Part model, mm, in its own coordinate system. A direction names the side the tool comes from. Round coordinates to 2 decimals unless told otherwise and drop trailing zeros. Order: outer loops, then holes, each group sorted by start corner. A loop starts at its lowest first (then second) coordinate and runs counter-clockwise, first axis right, second up. Notation, with made-up numbers: M 32.5,75 L 86.5,75 A31 cw 86.5,113 Z; hole C 17,-23 d3. An arc over 180 degrees is marked long. One line per question, with ' | ' between items.
Autodesk Inventor part; units mm, degrees
ref_plane "YZ Plane" through (0, 0, 0) normal (1, 0, 0) x (0, 1, 0)
ref_plane "XZ Plane" through (0, 0, 0) normal (0, 1, 0) x (-1, 0, 0)
ref_plane "XY Plane" through (0, 0, 0) normal (0, 0, 1) x (1, 0, 0)
sketch "スケッチ1" plane through (0, 0, 0) normal (0, 1, 0) x (-1, 0, 0)
  line L0 (25, -44) -> (-25, -44)
  line L1 (-25, -44) -> (-25, 44)
  line L2 (-25, 44) -> (25, 44)
  line L3 (25, 44) -> (25, -44)
  line L4 (25, -44) -> (-25, 44) construction
  line L5 (-25, -44) -> (25, 44) construction
  point P0 (0, 0)
  dimension "d0" = 50
  dimension "d1" = 88
extrude "押し出し1" add sketch "スケッチ1" against normal blind 2
sketch "スケッチ2" plane through (0, -2, 0) normal (0, -1, 0) x (1, 0, 0)
  line L0 (-25, 44) -> (-25, -44)
  line L1 (25, -44) -> (25, 44)
  line L2 (-25, -44) -> (25, -44)
  line L3 (25, -44) -> (25, -42)
  line L4 (25, -42) -> (-25, -42)
  line L5 (-25, -42) -> (-25, -44)
  line L6 (25, 44) -> (-25, 44)
  line L7 (-25, 44) -> (25, 44)
  line L8 (25, 44) -> (25, 42)
  line L9 (25, 42) -> (-25, 42)
  line L10 (-25, 42) -> (-25, 44)
  point P0 (0, 0)
  point P1 (-25, 42)
  point P2 (25, 42)
  point P3 (25, -44)
  dimension "d4" = 2
  dimension "d5" = 2
extrude "押し出し2" add sketch "スケッチ2" along normal blind 53 contours L6 L1 L9 L0 | L4 L1 L2 L0
sketch "スケッチ3" plane through (-25, 0, 44) normal (0, 0, 1) x (1, 0, 0)
  line L0 (0, 0) -> (50, 0)
  line L1 (0, 0) -> (0, -55)
  line L2 (50, -55) -> (0, -55)
  line L3 (50, 0) -> (50, -55)
  circle A0 centre (25, -30) radius 25
  line L4 (50, 0) -> (50, -55)
  point P0 (25, 0)
  point P1 (50, -30)
  point P2 (25, -55)
  point P3 (0, -30)
extrude "押し出し3" cut sketch "スケッチ3" against normal through all contours A0 L2 L1 | L3 L2 A0
move or copy body "移動1" bodies to move or copy 1 copy no translate (0, 30, 0)
sketch "スケッチ4" plane through (-25, 28, 42) normal (0, -1, 0) x (1, 0, 0)
  circle A0 centre (25, -42) radius 34
  dimension "d14" = 68
extrude "押し出し4" add sketch "スケッチ4" against normal blind 18
fillet "フィレット2" radius 12 4 edges at (25, 29, 23.0434) (25, 29, -23.0434) (-25, 29, 23.0434) (-25, 29, -23.0434)
properties part number "link4"
1) Saw through at D-D (y = 41.5). List the corners of the cut face in (x, z), plus the area to 3 significant figures.
The answers:
outline: C 0,0 d68 | area: 3,630 mm²
2) Drop flat-ended pins along their axis: pin 1 (1.5 mm diameter, centred on x = -9.5, z = -16.5, fed in from -Y); pin 2 (13.5 mm diameter, centred on y = 15.5, z = 38.5, fed in from -X); pin 3 (7 mm diameter, centred on x = -8.5, z = 37, fed in from +Y). Give the stop position or say it passes through.
The answers:
pin 1: stops at y = 28 | pin 2: stops at x = -25 | pin 3: stops at y = 30
3) Saw through at B-B (x = 0). List the corners of the cut face in (y, z).
The answers:
outline: M -25,-44 L 30,-44 L 30,-34 L 46,-34 L 46,34 L 30,34 L 30,44 L -25,44 L -25,42 L 28,42 L 28,-42 L -25,-42 Z
4) Saw through at C-C (z = -31). List the corners of the cut face in (x, y), plus the area to 3 significant figures.
The answers:
outline: M -25,28 L 25,28 L 25,30 L 13.96,30 L 13.96,46 L -13.96,46 L -13.96,30 L -25,30 Z | area: 547 mm²
5) Two-plate mould, pull along Z, no slides. Class faces 5 (the face through (0, 2, -42)), 6 (the face through (0, 2, 42)), 7 (the face through (0, 3, -44)), 8 (the face through (0, 30, 38)): released by +Z, released by -Z, zero draft, split by the parting line, or undercut.
The answers:
face 5: undercut | face 6: undercut | face 7: released by -Z | face 8: zero draft
6) Saw through at A-A (y = 26.5). List the corners of the cut face in (x, z), plus the area to 3 significant figures.
The answers:
outline: M -25,-44 L 25,-44 L 25,-42 L -25,-42 Z; M -25,42 L 25,42 L 25,44 L -25,44 Z | area: 200 mm²
7) Probe line 1 (Z direction, x = 23, y = -1); line 2 (Y direction, x = -24.5, z = 19); line 3 (Y direction, x = 8.5, z = -40). List the from-to ranges inside material, lowest first. Write a range as [from, to].
The answers:
line 1: z = [-44, -42], [42, 44] | line 2: y = [28, 46] | line 3: y = [28, 30]
8) Which spindle directions (+Z, -Z, +X, -X, +Y, -Y) get a long thin tool onto all of the face, cutting with end or side? Do faces 1 (the face through (25, 20.6, 42.4)), 2 (the face through (-25, 19.5, 42.5)), 3 (the face through (0, 30, -37)), 4 (the face through (25, 19.5, -42.5)). Say none if no direction does.
The answers:
face 1: +Z, +X, +Y, -Y | face 2: +Z, -X, +Y, -Y | face 3: -Z, +Y | face 4: -Z, +X, +Y, -Y
